Here's how the part is built. I have some questions about the finished solid (model axes, mm). A direction names the side the tool comes from. Round coordinates to 2 decimals unless told otherwise and drop trailing zeros. Loops run counter-clockwise (first coordinate to the right, second up) from the corner with the lowest first, then second, coordinate; pieces in that order, holes last. Notation, with made-up numbers: M -6,-1.5 L 14,-1.5 A14 cw 14,10.5 Z; hole C 21.25,-17.5 d8. An arc over 180 degrees is marked long. Answer as CSV lines item,"result".
```python
from build123d import *

# Parameters (mm, degrees)
SKETCH1_W           = 49.9999
SKETCH1_H           = 49.9999
SKETCH1_R           = 1.524
SKETCH1_R_2         = 1.27
BOSS_EXTRUDE1_DEPTH = 6.35
SKETCH2_R           = 3.81
CUT_EXTRUDE1_DEPTH  = 3.175


with BuildPart() as part:
    # Sketch1 → Boss-Extrude1 (new body)
    with BuildSketch(Plane(origin=(0, 0, 0), x_dir=(1, 0, 0), z_dir=(0, 1, 0))):
        with Locations((24.99995, 24.99995)):
            Rectangle(SKETCH1_W, SKETCH1_H)
        with Locations((4.9999392, 44.9999608)):
            Circle(SKETCH1_R, mode=Mode.SUBTRACT)
        with Locations((44.9999608, 44.9999608)):
            Circle(SKETCH1_R, mode=Mode.SUBTRACT)
        with Locations((44.9999608, 4.9999392)):
            Circle(SKETCH1_R, mode=Mode.SUBTRACT)
        with Locations((4.9999392, 4.9999392)):
            Circle(SKETCH1_R, mode=Mode.SUBTRACT)
        with Locations((14.9999446, 34.9999554)):
            Circle(SKETCH1_R_2, mode=Mode.SUBTRACT)
        with Locations((34.9999554, 34.9999554)):
            Circle(SKETCH1_R_2, mode=Mode.SUBTRACT)
        with Locations((34.9999554, 14.9999446)):
            Circle(SKETCH1_R_2, mode=Mode.SUBTRACT)
        with Locations((14.9999446, 14.9999446)):
            Circle(SKETCH1_R_2, mode=Mode.SUBTRACT)
    extrude(amount=BOSS_EXTRUDE1_DEPTH)

    # Sketch2 → Cut-Extrude1 (cut)
    with BuildSketch(Plane(origin=(0, 6.35, 0), x_dir=(1, 0, 0), z_dir=(0, 1, 0))):
        with Locations((4.9999392, 44.9999608)):
            Circle(SKETCH2_R)
        with Locations((44.9999608, 44.9999608)):
            Circle(SKETCH2_R)
        with Locations((4.9999392, 4.9999392)):
            Circle(SKETCH2_R)
        with Locations((44.9999608, 4.9999392)):
            Circle(SKETCH2_R)
    extrude(amount=-CUT_EXTRUDE1_DEPTH, mode=Mode.SUBTRACT)


solid = part.part
```
1. We'd pull the mould along Z, two halves only. Please class faces 1 (the cylindrical face through (34.83, 3.13, -36.26)), 2 (the flat face through (25, 3, -50)), 3 (the cylindrical face through (42.19, 4.78, -47.57)), 4 (the flat face through (50, 3, -25)): pulls with the +Z half, pulls with the -Z half, needs draft (parallel to the pull), parting line crosses it, or undercut.
Evaluation:
face 1,"undercut"
face 2,"pulls with the -Z half"
face 3,"undercut"
face 4,"needs draft"
2. I want a section at B-B, the plane y = 4.5. Count the separate pieces of the cut face and the enclosed holes in it, and give its area (3 significant figures).
Evaluation:
separate pieces,"1"
enclosed holes,"8"
area,"2,300 mm²"
3. Which directions (+Z, -Z, +X, -X, +Y, -Y) give clear straight access to the entire face, cutting with the end or side of a thin tool? Please do faces 5 (the flat face through (45, 3.175, -3)), 6 (the cylindrical face through (33.73, 3.13, -15.06)).
Evaluation:
face 5,"+Y"
face 6,"+Y, -Y"
4. I want a section at A-A, the plane x = 5. Please give me the cut outline in (y, z) (3 decimals), and give its area (3 significant figures).
Evaluation:
outline,"M 0,-50 L 6.35,-50 L 6.35,-48.81 L 3.175,-48.81 L 3.175,-46.524 L 0,-46.524 Z; M 0,-43.476 L 3.175,-43.476 L 3.175,-41.19 L 6.35,-41.19 L 6.35,-8.81 L 3.175,-8.81 L 3.175,-6.524 L 0,-6.524 Z; M 0,-3.476 L 3.175,-3.476 L 3.175,-1.19 L 6.35,-1.19 L 6.35,0 L 0,0 Z"
area,"250 mm²"
5. If I drill on line 1 (Z direction, x = 47.5, y = 6) (3 decimals); line 2 (X direction, y = 4.75, z = -7); line 3 (Z direction, x = 44.5, y = 2.75), over which ranges is the centre line in solid material (lowest first)? Write a range as [from, to].
Evaluation:
line 1,"z = [-50, -47.875], [-42.125, -7.875], [-2.125, 0]"
line 2,"x = [0, 1.76], [8.24, 41.76], [48.24, 50]"
line 3,"z = [-50, -46.44], [-43.56, -6.44], [-3.56, 0]"
6. For P1, Ø2.5, axis at x = 46, z = -47, coming from the +Y side (3 decimals), with a flat end and sliding along its axis, tell me the tip position at first contact or that it passes through.
Evaluation:
P1,"stops at y = 3.175"
7. I want a section at C-C, the plane x = 47.5. Please give me the cut outline in (y, z) (3 decimals).
Evaluation:
outline,"M 0,-50 L 6.35,-50 L 6.35,-47.875 L 3.175,-47.875 L 3.175,-42.125 L 6.35,-42.125 L 6.35,-7.875 L 3.175,-7.875 L 3.175,-2.125 L 6.35,-2.125 L 6.35,0 L 0,0 Z"
